Check sheet for the modelled part. Datum: model origin and axes. Units: mm. A direction names the side the tool comes from. Round coordinates to 2 decimals unless told otherwise and drop trailing zeros. Order: outer loops, then holes, each group sorted by start corner. A loop starts at its lowest first (then second) coordinate and runs counter-clockwise, first axis right, second up.
```python
from build123d import *

# Parameters (mm, degrees)
CUT_EXTRUDE1_DEPTH = 10
CIRPATTERN1_COUNT  = 32


with BuildPart() as part:
    # Sketch1 → Revolve1 (revolve)
    with BuildSketch(Plane(origin=(0, 0, 0), x_dir=(1, 0, 0), z_dir=(0, 1, 0)), mode=Mode.PRIVATE) as revolve1_sk:
        Polygon((1, 0), (6.5, 0), (6.5, 2), (7.5, 2), (7.5, -1), (2.5, -1), (2.5, -4), (1, -4), align=None)
    revolve(revolve1_sk.sketch.rotate(Axis((0, 0, -10.710116732), (0, 0, 1)), 180), axis=Axis((0, 0, -10.710116732), (0, 0, 1)))

    # Sketch2 → Cut-Extrude1 (cut)
    with BuildSketch(Plane(origin=(0, 0, 0), x_dir=(1, 0, 0), z_dir=(0, 1, 0))):
        Polygon((0, 1.284275778), (2.060090555, 3.344366332), (-2.060090555, 3.344366332), align=None)
    cut_extrude1 = extrude(amount=-CUT_EXTRUDE1_DEPTH, mode=Mode.SUBTRACT)

    # CirPattern1: Cut-Extrude1 ×32 about axis
    cirpattern1_axis = Axis((0, 0, 0), (0, 0, 1))
    for i in range(1, CIRPATTERN1_COUNT):
        add(cut_extrude1.rotate(cirpattern1_axis, i * 360 / CIRPATTERN1_COUNT), mode=Mode.SUBTRACT)


solid = part.part
```
Item 1: Access from +Z, -Z, +X, -X, +Y, -Y to the whole of each face (thin tool, end or side, straight path). Record for faces 4 (the flat face through (-6.31, 3.01, -1.65)), 5 (the cylindrical face through (0, 1, 2)).
Answer:
face 4: -Z
face 5: +Z, -Z
Item 2: Release check for a two-part mould opening along X. For faces 1 (the flat face through (-4.18, -5.6, -1.65)), 2 (the flat face through (-1, 1, 4)), 3 (the cylindrical face through (2.5, -0.1, 2.5)) record: released by +X, released by -X, zero draft, split by the parting line, or undercut.
Answer:
face 1: undercut
face 2: zero draft
face 3: split by the parting line
Item 3: Scan lines: line 1 along Y through (x, z) = (0, -0.5); line 2 along Y through (x, z) = (-5, -1.5); line 3 along Z through (x, y) = (-1.75, 4.5). Record each from-to range of solid material in increasing order.
Answer:
line 1: y = -7.5 to -6.5, 6.5 to 7.5
line 2: y = -5.59 to -5.31, -4.69 to -4.15, 4.15 to 4.69, 5.31 to 5.59
line 3: z = 0 to 1
Item 4: Go/stop test with flat-tipped pins: P1, Ø3, axis at x = 4, y = 0, coming from the -Z side; P2, Ø1.5, axis at y = -1.5, z = 3, coming from the -X side. Record where each tip stops, or that it passes through.
Answer:
P1: stops at z = 0
P2: stops at x = -2.38
Item 5: Sectioned sample at B-B (z = -1.5). State how many separate pieces and enclosed holes the cut face has, and give its area (3 significant figures).
Answer:
separate pieces: 32
enclosed holes: 0
area: 30.2 mm2
Item 6: Sectioned sample at C-C (z = 0.5). Record the cut outline in (x, y).
Answer:
outline: circle Ø15 at (0, 0); hole circle Ø2 at (0, 0)
Item 7: Sectioned sample at A-A (z = 2.75). Record the cut outline in (x, y), and give its area (3 significant figures).
Answer:
outline: circle Ø5 at (0, 0); hole circle Ø2 at (0, 0)
area: 16.5 mm2
